Design review of the part built by this model. Coordinates are the model's own, in mm. A direction names the side the tool comes from. Round coordinates to 2 decimals unless told otherwise and drop trailing zeros. Write each loop counter-clockwise with the first axis right and the second up, starting at its lowest first coordinate (ties: lowest second). Pieces come first, ordered by that corner, then holes.
from build123d import *

# Parameters (mm, degrees)
SKETCH1_R               = 4.826
BOSS_EXTRUDE1_DEPTH     = 6.35
SKETCH2_R               = 31.75
SKETCH2_R_2             = 28.575
BOSS_EXTRUDE2_DEPTH     = 1209.802
BOSS_EXTRUDE3_START     = -25.4
SKETCH3_R               = 28.575
SKETCH3_R_2             = 25.4
BOSS_EXTRUDE3_DEPTH     = 25.4
CUT_EXTRUDE1_DEPTH      = 6.35
CUT_EXTRUDE1_DEPTH_BACK = 6.35
FILLET1_ANGLE           = 290


with BuildPart() as part:
    # Sketch1 → Boss-Extrude1 (new body)
    with BuildSketch(Plane(origin=(0, 0, 0), x_dir=(1, 0, 0), z_dir=(0, 1, 0))):
        with BuildLine():
            Line((-46.814539331, 32.779893337), (0, 0))
            Line((0, 0), (-46.814539331, -32.779893337))
            ThreePointArc((-46.814539331, -32.779893337), (57.15, 0), (-46.814539331, 32.779893337))
        make_face()
        with Locations(Location((44.45, 0, 0), (0, 0, 270))):
            Circle(SKETCH1_R, mode=Mode.SUBTRACT)
        with Locations(Location((22.225, -38.494829198, 0), (0, 0, 270))):
            Circle(SKETCH1_R, mode=Mode.SUBTRACT)
        with Locations(Location((-22.225, -38.494829198, 0), (0, 0, 270))):
            Circle(SKETCH1_R, mode=Mode.SUBTRACT)
        with Locations(Location((-22.225, 38.494829198, 0), (0, 0, 270))):
            Circle(SKETCH1_R, mode=Mode.SUBTRACT)
        with Locations(Location((22.225, 38.494829198, 0), (0, 0, 270))):
            Circle(SKETCH1_R, mode=Mode.SUBTRACT)
    extrude(amount=BOSS_EXTRUDE1_DEPTH)

    # Sketch2 → Boss-Extrude2 (add)
    with BuildSketch(Plane(origin=(0, 6.35, 0), x_dir=(1, 0, 0), z_dir=(0, 1, 0))):
        with Locations(Location((0, 0, 0), (0, 0, 145))):
            Circle(SKETCH2_R)
        with Locations(Location((0, 0, 0), (0, 0, 145))):
            Circle(SKETCH2_R_2, mode=Mode.SUBTRACT)
    extrude(amount=BOSS_EXTRUDE2_DEPTH)

    # Sketch3 → Boss-Extrude3 (add)
    with BuildSketch(Plane(origin=(0, 1216.152, 0), x_dir=(1, 0, 0), z_dir=(0, 1, 0)).offset(BOSS_EXTRUDE3_START)):
        with Locations(Location((0, 0, 0), (0, 0, 145))):
            Circle(SKETCH3_R)
        with Locations(Location((0, 0, 0), (0, 0, 270))):
            Circle(SKETCH3_R_2, mode=Mode.SUBTRACT)
    extrude(amount=BOSS_EXTRUDE3_DEPTH)

    # Sketch4 → Cut-Extrude1 (cut, two sides: drawn at the far end of the back side and taken through both)
    with BuildSketch(Plane(origin=(13.5255, 0, -23.426853198), x_dir=(-0.8660254037844382, 0, -0.5000000000000009), z_dir=(0.5000000000000009, 0, -0.8660254037844382)).offset(-CUT_EXTRUDE1_DEPTH_BACK)):
        with BuildLine():
            Line((4.7625, 1185.9895), (4.7625, 712.9145))
            ThreePointArc((4.7625, 712.9145), (0, 708.152), (-4.7625, 712.9145))
            Line((-4.7625, 712.9145), (-4.7625, 1185.9895))
            ThreePointArc((-4.7625, 1185.9895), (0, 1190.752), (4.7625, 1185.9895))
        make_face()
    extrude(amount=CUT_EXTRUDE1_DEPTH + CUT_EXTRUDE1_DEPTH_BACK, mode=Mode.SUBTRACT)

    # Fillet1: read off the stored shape, not the designer's step
    # Fillet1 outline → Fillet1 (revolve)
    with BuildSketch(Plane(origin=(0, 0, 0), x_dir=(-0.8191520442889906, 0, 0.5735764363510478), z_dir=(-0.5735764363510478, 0, -0.8191520442889906))):
        with BuildLine():
            ThreePointArc((36.83, 6.35), (33.237897552, 7.837897552), (31.75, 11.43))
            Line((31.75, 11.43), (31.75, 6.35))
            Line((31.75, 6.35), (36.83, 6.35))
        make_face()
    revolve(axis=Axis((0, 0, 0), (0, 1, 0)), revolution_arc=FILLET1_ANGLE)


solid = part.part
1) For line 1 along Y through (x, z) = (-1, -28); line 2 along X through (y, z) = (891, 0) (3 decimals); line 3 along X through (y, z) = (361.5, -2), list the stretches that pass through material, from the lowest coordinate up.
2) For P1, Ø3, axis at x = -1.5, y = 619.5, coming from the +Z side; P2, Ø6.5, axis at x = -26, z = 7.5, coming from the -Y side; P3, Ø12, axis at x = 29.5, y = 1067, coming from the +Z side; P4, Ø7.5, axis at x = 22.22, z = -38.49, coming from the +Y side, all flat-tipped, find the tip position at first contact; note any pin that passes through.
3) For faces 1 (the face through (2, 6.35, 0)), 2 (the face through (-30.277, 602.782, -9.558)), 3 (the face through (-1, 1216.152, 26)), list the 3-axis set-ups (+Z, -Z, +X, -X, +Y, -Y) from which the entire face can be reached by the end or side of a thin tool; tool diameter is ignored.
4) Add section A-A on y = 536. State the section outline as (x, z) points (3 decimals), and give its area (3 significant figures).
5) The part is to be moulded in two halves that separate along Y. For faces 4 (the face through (28.55, 590.26, -1.24)), 5 (the face through (4, 0, -1)), 6 (the face through (25.4, 1190.752, -2.8)), 7 (the face through (39, 6.35, -1)), say which applies: pulls with the +Y half, pulls with the -Y half, needs draft (parallel to the pull), parting line crosses it, or undercut.
Computed:
1. line 1: y = 0 to 6.35, 1190.75 to 1216.15
1. line 2: x = -31.75 to -28.575, 28.575 to 31.75
1. line 3: x = -31.69 to -28.5, 28.5 to 31.69
2. P1: stops at z = 31.75
2. P2: stops at y = 6.35
2. P3: stops at z = 21.35
2. P4: passes through
3. face 1: none
3. face 2: +Y
3. face 3: +Z, -Z, +X, -X, +Y
4. outline: circle Ø63.5 at (0, 0); hole circle Ø57.15 at (0, 0)
4. area: 602 mm2
5. face 4: undercut
5. face 5: pulls with the -Y half
5. face 6: undercut
5. face 7: pulls with the +Y half
